Verification items for the finished model (mm, model axes). Face numbers are marked on the shaded views. A direction names the side the tool comes from. Round coordinates to 2 decimals unless told otherwise and drop trailing zeros. Order: outer loops, then holes, each group sorted by start corner. A loop starts at its lowest first (then second) coordinate and runs counter-clockwise, first axis right, second up.
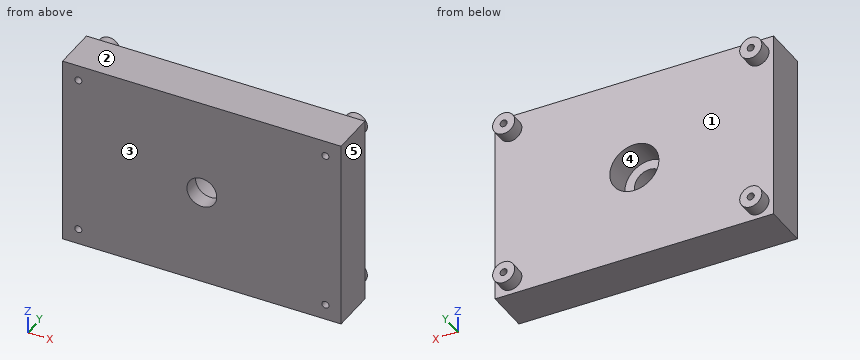
```python
from build123d import *

# Parameters (mm, degrees)
SKETCH1_W                                        = 63
SKETCH1_H                                        = 43
BOSS_EXTRUDE1_DEPTH                              = 10
CBORE_FOR_1_4_SOCKET_HEAD_CAP_SCREW1_D           = 6.7564
CBORE_FOR_1_4_SOCKET_HEAD_CAP_SCREW1_CBORE_D     = 11.1125
CBORE_FOR_1_4_SOCKET_HEAD_CAP_SCREW1_CBORE_DEPTH = 6.35
SKETCH6_R                                        = 2.5
BOSS_EXTRUDE2_DEPTH                              = 3
M2X0_4_TAPPED_HOLE1_D                            = 1.6


with BuildPart() as part:
    # Sketch1 → Boss-Extrude1 (new body)
    with BuildSketch(Plane(origin=(0, 0, 0), x_dir=(1, 0, 0), z_dir=(0, 1, 0))):
        Rectangle(SKETCH1_W, SKETCH1_H)
    extrude(amount=BOSS_EXTRUDE1_DEPTH)

    # CBORE for 1/4 Socket Head Cap Screw1 (through all)
    with Locations(Plane(origin=(0, 10, 0), x_dir=(1, 0, 0), z_dir=(0, 1, 0))):
        with Locations((0, 0)):
            CounterBoreHole(CBORE_FOR_1_4_SOCKET_HEAD_CAP_SCREW1_D / 2, CBORE_FOR_1_4_SOCKET_HEAD_CAP_SCREW1_CBORE_D / 2, CBORE_FOR_1_4_SOCKET_HEAD_CAP_SCREW1_CBORE_DEPTH)

    # Sketch6 → Boss-Extrude2 (add)
    with BuildSketch(Plane(origin=(0, 10, 0), x_dir=(1, 0, 0), z_dir=(0, 1, 0))):
        with Locations(Location((-27.95, 18, 0), (0, 0, 90))):
            Circle(SKETCH6_R)
        with Locations(Location((27.95, 18, 0), (0, 0, 90))):
            Circle(SKETCH6_R)
        with Locations(Location((27.95, -18, 0), (0, 0, 90))):
            Circle(SKETCH6_R)
        with Locations(Location((-27.95, -18, 0), (0, 0, 90))):
            Circle(SKETCH6_R)
    extrude(amount=BOSS_EXTRUDE2_DEPTH)

    # M2x0.4 Tapped Hole1 (through all)
    with Locations(Plane(origin=(0, 13, 0), x_dir=(1, 0, 0), z_dir=(0, 1, 0))):
        with Locations((-27.95, 18), (27.95, 18), (27.95, -18), (-27.95, -18)):
            Hole(M2X0_4_TAPPED_HOLE1_D / 2)


solid = part.part
```
1) Sectioned sample at D-D on y = 4.5. Record the cut outline in (x, z), then the cut area to 3 significant figures.
2) Sectioned sample at B-B on x = 27.95. Record the cut outline in (y, z).
3) Sectioned sample at A-A on y = 11.5. Record the cut outline in (x, z), then the cut area to 3 significant figures.
4) Tool access check on the marked faces 1 and 2. Record the directions out of +Z, -Z, +X, -X, +Y, -Y that give a thin tool (end or side, any length) a straight path to the whole face; none if there is none.
5) Draft check along X on the marked faces 3, 4 and 5. Enter one of: released by +X, released by -X, zero draft, split by the parting line, or undercut.
6) Go/stop test with flat-tipped pins: pin 1 Ø21.5 at (x, z) = (14, -3.5) entering from +Y; pin 2 Ø3.5 at (x, z) = (0.5, -2) entering from +Y. Record where each tip stops, or that it passes through.
7) Scan lines: probe 1 along X at (y, z) = (6, 18); probe 2 along Z at (x, y) = (-27.95, 8.5); probe 3 along X at (y, z) = (5.5, 17.5). Record each from-to range of solid material in increasing order.
8) Sectioned sample at C-C on z = -18. Record the cut outline in (x, y), then the cut area to 3 significant figures.
Returned:
1. outline: (-31.5, -21.5) - (31.5, -21.5) - (31.5, 21.5) - (-31.5, 21.5) - close; hole circle Ø1.6 at (-27.95, -18); hole circle Ø1.6 at (-27.95, 18); hole circle Ø11.11 at (0, 0); hole circle Ø1.6 at (27.95, -18); hole circle Ø1.6 at (27.95, 18)
1. area: 2,600 mm2
2. outline: (0, -21.5) - (10, -21.5) - (10, -20.5) - (13, -20.5) - (13, -18.8) - (0, -18.8) - close; (0, -17.2) - (13, -17.2) - (13, -15.5) - (10, -15.5) - (10, 15.5) - (13, 15.5) - (13, 17.2) - (0, 17.2) - close; (0, 18.8) - (13, 18.8) - (13, 20.5) - (10, 20.5) - (10, 21.5) - (0, 21.5) - close
3. outline: circle Ø5 at (-27.95, -18); circle Ø5 at (-27.95, 18); circle Ø5 at (27.95, -18); circle Ø5 at (27.95, 18); hole circle Ø1.6 at (-27.95, -18); hole circle Ø1.6 at (-27.95, 18); hole circle Ø1.6 at (27.95, -18); hole circle Ø1.6 at (27.95, 18)
3. area: 70.5 mm2
4. face 1: +Y
4. face 2: +Z, +X, -X, +Y, -Y
5. face 3: zero draft
5. face 4: undercut
5. face 5: released by +X
6. pin 1: stops at y = 10
6. pin 2: stops at y = 3.65
7. probe 1: x = -31.5 to -28.75, -27.15 to 27.15, 28.75 to 31.5
7. probe 2: z = -21.5 to -18.8, -17.2 to 17.2, 18.8 to 21.5
7. probe 3: x = -31.5 to -28.57, -27.33 to 27.33, 28.57 to 31.5
8. outline: (-31.5, 0) - (-28.75, 0) - (-28.75, 13) - (-30.45, 13) - (-30.45, 10) - (-31.5, 10) - close; (-27.15, 0) - (27.15, 0) - (27.15, 13) - (25.45, 13) - (25.45, 10) - (-25.45, 10) - (-25.45, 13) - (-27.15, 13) - close; (28.75, 0) - (31.5, 0) - (31.5, 10) - (30.45, 10) - (30.45, 13) - (28.75, 13) - close
8. area: 618 mm2
